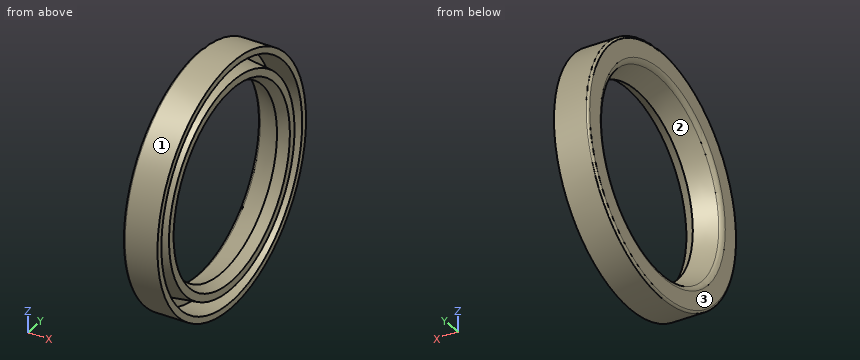
from build123d import *


with BuildPart() as part:
    # Sketch1 → Revolve2 (revolve)
    with BuildSketch(Plane.XY):
        with BuildLine():
            Line((0.9025, 9.714192053), (0.9025, 8.997599754))
            Line((0.9025, 8.997599754), (0.005, 8.5))
            Line((0.005, 8.5), (0, 8.5))
            Line((0, 8.5), (-1.96898625, 9.218913515))
            ThreePointArc((-1.96898625, 9.218913515), (-2.207221323, 9.402005642), (-2.2975, 9.688586237))
            Line((-2.2975, 9.688586237), (-2.2975, 11.3))
            ThreePointArc((-2.2975, 11.3), (-2.238921356, 11.441421356), (-2.0975, 11.5))
            Line((-2.0975, 11.5), (0.9025, 11.5))
            Line((0.9025, 11.5), (0.9025, 10.9))
            Line((0.9025, 10.9), (-1.6975, 10.9))
            Line((-1.6975, 10.9), (-1.6975, 10.039192053))
            Line((-1.6975, 10.039192053), (0.9025, 9.714192053))
        make_face()
    revolve(axis=Axis((0, 0, 0), (-1, 0, 0)))


solid = part.part
Model file for the job. Use its own axes, mm. Face numbers are marked on the shaded views. Give positions to 0.01 mm unless a question says otherwise; leave off trailing zeros. Loops run counter-clockwise (first coordinate to the right, second up) from the corner with the lowest first, then second, coordinate; pieces in that order, holes last.
1) Flat gauge pin, fed straight in: pin 1 Ø3 at (y, z) = (-5.5, 4.5) entering from +X. Where does the tip first touch, or does it go through?
2) Wall check: line 1 (Z direction, x = 0, y = 0); line 2 (Z direction, x = -0.5, y = 0); line 3 (Y direction, x = -1.05, z = -4). Give the ranges that are in metal, low to high.
3) Pull direction Z, two halves, no side cores. Call the marked faces 1, 2 and 3: +Z half, -Z half, draft (parallel to the pull), parting line (faces both ways), or undercut.
4) Saw through at C-C (x = -1). Write the cut outline in (y, z).
Answer block:
1. pin 1: stops at x = 0.2
2. line 1: z = -11.5 to -10.9, -9.83 to -8.5, 8.5 to 9.83, 10.9 to 11.5
2. line 2: z = -11.5 to -10.9, -9.89 to -8.68, 8.68 to 9.89, 10.9 to 11.5
2. line 3: y = -10.78 to -10.14, -9.12 to -7.93, 7.93 to 9.12, 10.14 to 10.78
3. face 1: parting line
3. face 2: undercut
3. face 3: draft
4. outline: circle Ø23 at (0, 0); circle Ø19.9 at (0, 0); hole circle Ø21.8 at (0, 0); hole circle Ø17.73 at (0, 0)
